Can you work these out from the drawing? Everything is in mm from the part's minimum corner. A direction names the side the tool comes from. Give positions to 0.01 mm unless a question says otherwise; leave off trailing zeros. Order: outer loops, then holes, each group sorted by start corner. A loop starts at its lowest first (then second) coordinate and runs counter-clockwise, first axis right, second up. Notation, with made-up numbers: M -39.75,-0.5 L 0.25,-0.5 A24 cw 0.25,28.5 Z; hole C 36,33 d2. An arc over 180 degrees is marked long. Answer as a JSON object with one key per item and string values.
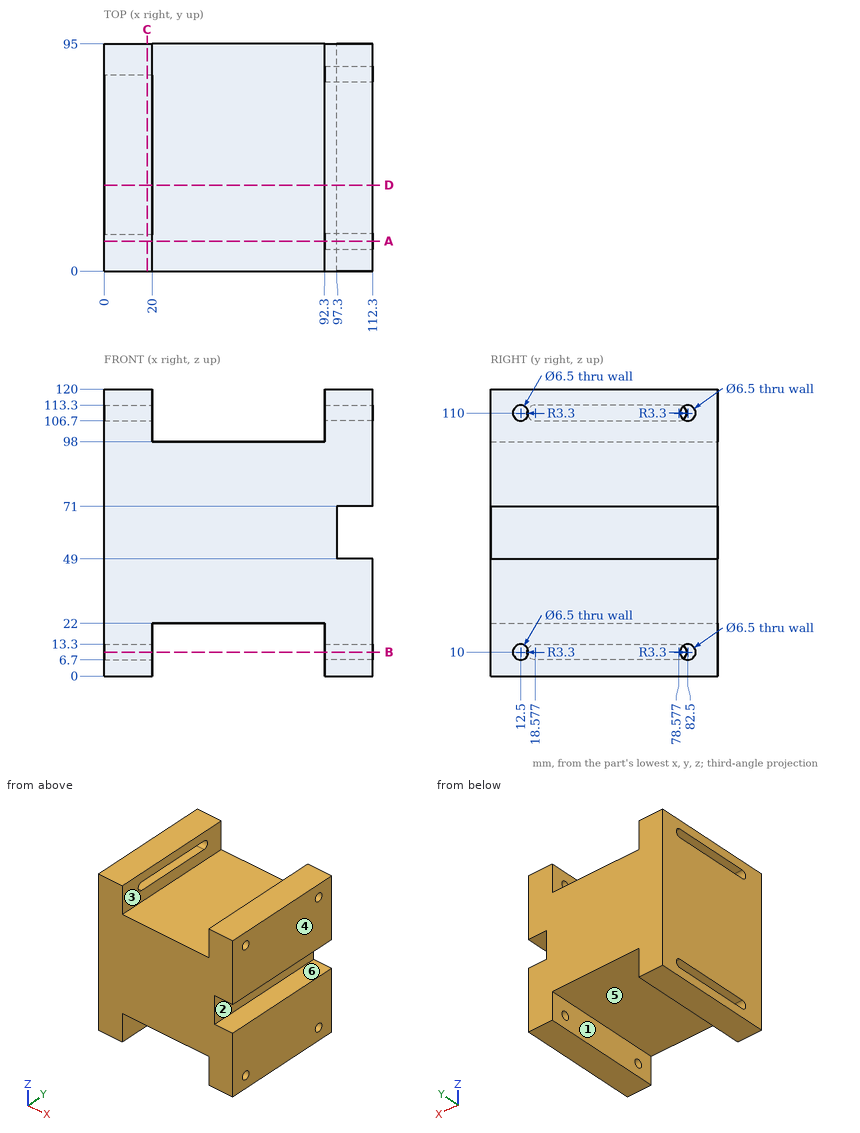
1) I need wall thicknesses on L1, parallel to Y at x = 103, z = 110; L2, parallel to Z at x = 12.5, y = 18; L3, parallel to X at y = 28, z = 16.5. Which ranges of each line are inside material? Lowest first, please.
Results found:
{"L1": "y = 0 to 9.25, 15.75 to 79.25, 85.75 to 95", "L2": "z = 0 to 6.75, 13.25 to 106.75, 113.25 to 120", "L3": "x = 0 to 20, 92.3 to 112.3"}
2) For the marked faces 1, 2 and 3, which set-ups out of +Z, -Z, +X, -X, +Y, -Y let a thin tool reach every point of the face, with its end or its side?
Results found:
{"face 1": "-Z, +Y, -Y", "face 2": "+X, +Y, -Y", "face 3": "+Z, +Y, -Y"}
3) I want a section at B-B on z = 10. Write out the boundary of the cut face in (x, y), and give its area (3 significant figures).
Results found:
{"outline": "M 0,0 L 20,0 L 20,15.28 L 0,15.28 Z; M 0,81.88 L 20,81.88 L 20,95 L 0,95 Z; M 92.3,0 L 112.3,0 L 112.3,9.25 L 92.3,9.25 Z; M 92.3,15.75 L 112.3,15.75 L 112.3,79.25 L 92.3,79.25 Z; M 92.3,85.75 L 112.3,85.75 L 112.3,95 L 92.3,95 Z", "area": "2,210 mm²"}
4) Thinking about a two-plate mould opening in Z: for the marked faces 4, 5 and 6, which applies, pulls with the +Z half, pulls with the -Z half, needs draft (parallel to the pull), parting line crosses it, or undercut?
Results found:
{"face 4": "needs draft", "face 5": "pulls with the -Z half", "face 6": "undercut"}
5) I want a section at A-A on y = 12.5. Write out the boundary of the cut face in (x, z).
Results found:
{"outline": "M 0,0 L 20,0 L 20,22 L 92.3,22 L 92.3,13.25 L 112.3,13.25 L 112.3,49 L 97.3,49 L 97.3,71 L 112.3,71 L 112.3,106.75 L 92.3,106.75 L 92.3,98 L 20,98 L 20,120 L 0,120 Z; M 92.3,0 L 112.3,0 L 112.3,6.75 L 92.3,6.75 Z; M 92.3,113.25 L 112.3,113.25 L 112.3,120 L 92.3,120 Z"}
6) I'm going to push flat-ended pins straight in: pin 1 Ø4 at (y, z) = (13, 65) entering from +X; pin 2 Ø1 at (x, y) = (37, 59.5) entering from -Z; pin 3 Ø10 at (x, y) = (71, 18.5) entering from +Z. Where does each tip first touch, or does it pass through?
Results found:
{"pin 1": "stops at x = 97.3", "pin 2": "stops at z = 22", "pin 3": "stops at z = 98"}
7) I want a section at C-C on x = 18. Write out the boundary of the cut face in (y, z), and give its area (3 significant figures).
Results found:
{"outline": "M 0,0 L 95,0 L 95,120 L 0,120 Z; hole M 18.58,6.7 L 78.58,6.7 A3.3 ccw 78.58,13.3 L 18.58,13.3 A3.3 ccw Z; hole M 18.58,106.7 L 78.58,106.7 A3.3 ccw 78.58,113.3 L 18.58,113.3 A3.3 ccw Z", "area": "10,500 mm²"}
8) I want a section at D-D on y = 36. Write out the boundary of the cut face in (x, z), and give its area (3 significant figures).
Results found:
{"outline": "M 0,0 L 20,0 L 20,6.7 L 0,6.7 Z; M 0,13.3 L 20,13.3 L 20,22 L 92.3,22 L 92.3,0 L 112.3,0 L 112.3,49 L 97.3,49 L 97.3,71 L 112.3,71 L 112.3,120 L 92.3,120 L 92.3,98 L 20,98 L 20,106.7 L 0,106.7 Z; M 0,113.3 L 20,113.3 L 20,120 L 0,120 Z", "area": "9,700 mm²"}
